Check sheet for the modelled part. Datum: model origin and axes. Units: mm. A direction names the side the tool comes from. Give positions to 0.01 mm unless a question says otherwise; leave off trailing zeros. Order: outer loops, then holes, each group sorted by start corner. A loop starts at its lowest first (then second) coordinate and runs counter-clockwise, first axis right, second up. Notation, with made-up numbers: (82.5, 59) - (119.5, 59) arc R33 ccw to (119.5, 96) - close; hole circle Ø4 at (-33.5, 16.5). An arc over 180 degrees is marked (long way). Answer in a Markdown table with one row per item.
from build123d import *

# Parameters (mm, degrees)
F1_DEPTH = 50.8


with BuildPart() as f1:
    # F0 (on Top) → F1 (new body)
    with BuildSketch(Plane.XY):
        with BuildLine():
            Line((-52.733865, 0), (0, 0))
            Line((0, 0), (0, 181.136057))
            ThreePointArc((0, 181.136057), (-17.94511, 169.62391), (-28.517708, 151.109681))
            Line((-28.517708, 151.109681), (-41.49279, 105.66102))
            Line((-41.49279, 105.66102), (-41.49279, 37.194733))
            Line((-41.49279, 37.194733), (-52.733865, 14.051343))
            Line((-52.733865, 14.051343), (-52.733865, 0))
        make_face()
    extrude(amount=F1_DEPTH)


solid = f1.part
(1) Cross-section at B-B, the plane y = 63. Record the cut outline in (x, z), then the cut area to 3 significant figures.
Geometry says:
| item | result |
|---|---|
| outline | (-41.49, 0) - (0, 0) - (0, 50.8) - (-41.49, 50.8) - close |
| area | 2,110 mm² |
(2) Cross-section at A-A, the plane z = 19. Record the cut outline in (x, y).
Geometry says:
| item | result |
|---|---|
| outline | (-52.73, 0) - (0, 0) - (0, 181.14) arc R44.71 ccw to (-28.52, 151.11) - (-41.49, 105.66) - (-41.49, 37.19) - (-52.73, 14.05) - close |
(3) Gauge pin test, flat ends, axial feed: P1, Ø4, axis at x = -44, z = 7.5, coming from the +Y side; P2, Ø8, axis at x = -18.5, z = 31.5, coming from the +Y side; P3, Ø10, axis at x = -6, z = 40.5, coming from the +Y side. Record the tip position at first contact, or that the pin passes through.
Geometry says:
| item | result |
|---|---|
| P1 | y = 36.15 |
| P2 | y = 172.89 |
| P3 | y = 180.78 |
(4) Cross-section at C-C, the plane x = -13.5. Record the cut outline in (y, z).
Geometry says:
| item | result |
|---|---|
| outline | (0, 0) - (173.71, 0) - (173.71, 50.8) - (0, 50.8) - close |
(5) Thickness scan on L1, parallel to X at y = 58, z = 24; L2, parallel to Y at x = -23, z = 5; L3, parallel to Y at x = -22.5, z = 45. Record the ranges inside material, lowest first.
Geometry says:
| item | result |
|---|---|
| L1 | -41.49 to 0 |
| L2 | 0 to 163.22 |
| L3 | 0 to 163.97 |
(6) Access from +Z, -Z, +X, -X, +Y, -Y to the whole of each face (thin tool, end or side, straight path). Record for faces 1 (the flat face through (-41.493, 72, 25)), 2 (the flat face through (-21, 72, 0)).
Geometry says:
| item | result |
|---|---|
| face 1 | +Z, -Z, -X, +Y |
| face 2 | -Z, +X, -X, +Y, -Y |
